Work out the finished part from the listing and answer in its coordinate system (mm). Coordinates: 2 decimals unless noted, no trailing zeros. Loops run counter-clockwise (first coordinate to the right, second up) from the corner with the lowest first, then second, coordinate; pieces in that order, holes last. Notation, with made-up numbers: (87, 44) - (141, 44) arc R29 ccw to (141, 67) - close; hole circle Ø9 at (-3, -4). An arc over 180 degrees is marked (long way). Write each question's results on one line, items separated by ' | '. Start each with the question number.
1. Find the intervals of material crossed by line 1 along X through (y, z) = (1.15, 17.5); line 2 along X through (y, z) = (0.75, 2); line 3 along Z through (x, y) = (20, 2.25), in increasing order. Write a range as [from, to].
2. A cutting plane is placed at B-B on y = 1.8. Determine the outline of the cut face in (x, z).
3. A cutting plane is placed at D-D on z = -17. Determine the outline of the cut face in (x, y).
4. A cutting plane is placed at A-A on z = 17.5. Determine the outline of the cut face in (x, y).
5. A cutting plane is placed at C-C on x = -20. Determine the outline of the cut face in (y, z).
6. This flat-tipped pin is pushed along its axis until it touches: P1, Ø0.9, axis at x = 20.5, y = 1.5, coming from the -Z side. Where does it stop, or does it pass through?
from build123d import *

# Parameters (mm, degrees)
SKETCH_1_W          = 50
SKETCH_1_H          = 55
EXTRUDE_1_DEPTH     = 3
SKETCH_2_R          = 4
CUT_EXTRUDE_1_DEPTH = 3
SKETCH_3_R          = 2
CUT_EXTRUDE_2_DEPTH = 3
SKETCH_4_W          = 3
SKETCH_4_H          = 10
CUT_EXTRUDE_3_DEPTH = 3
CHAMFER_1_SIZE      = 30
CHAMFER_1_SIZE2     = 21.006226146
FILLET_2_R          = 10
FILLET_3_R          = 5


with BuildPart() as part:
    # 草图1 → 凸台-拉伸1 (new body)
    with BuildSketch(Plane(origin=(0, 0, 0), x_dir=(1, 0, 0), z_dir=(0, 1, 0))):
        Rectangle(SKETCH_1_W, SKETCH_1_H)
    extrude(amount=EXTRUDE_1_DEPTH)

    # 草图2 → 切除-拉伸1 (cut)
    with BuildSketch(Plane(origin=(0, 3, 0), x_dir=(1, 0, 0), z_dir=(0, 1, 0))):
        with Locations(Location((4, 17, 0), (0, 0, 270))):
            Circle(SKETCH_2_R)
    extrude(amount=-CUT_EXTRUDE_1_DEPTH, mode=Mode.SUBTRACT)

    # 草图3 → 切除-拉伸2 (cut)
    with BuildSketch(Plane(origin=(0, 3, 0), x_dir=(1, 0, 0), z_dir=(0, 1, 0))):
        with Locations(Location((-20, -17.5, 0), (0, 0, 270))):
            Circle(SKETCH_3_R)
        with Locations(Location((0, -17.5, 0), (0, 0, 270))):
            Circle(SKETCH_3_R)
        with Locations(Location((20, -17.5, 0), (0, 0, 90))):
            Circle(SKETCH_3_R)
    extrude(amount=-CUT_EXTRUDE_2_DEPTH, mode=Mode.SUBTRACT)

    # 草图4 → 切除-拉伸3 (cut)
    with BuildSketch(Plane(origin=(0, 3, 0), x_dir=(1, 0, 0), z_dir=(0, 1, 0))):
        with Locations((-20.5, -2.5)):
            Rectangle(SKETCH_4_W, SKETCH_4_H)
        with Locations((20.5, -2.5)):
            Rectangle(SKETCH_4_W, SKETCH_4_H)
        with Locations((20.5, 17.5)):
            Rectangle(SKETCH_4_W, SKETCH_4_H)
    extrude(amount=-CUT_EXTRUDE_3_DEPTH, mode=Mode.SUBTRACT)

    # 倒角1
    chamfer_1_edges = [part.edges().sort_by_distance(p)[0] for p in [
        (-25, 1.5, -27.5),
    ]]
    chamfer_1_side = [part.faces().sort_by_distance(p)[0] for p in [
        (0, 1.5, -27.5),
    ]]
    chamfer(chamfer_1_edges, length=CHAMFER_1_SIZE, length2=CHAMFER_1_SIZE2, reference=chamfer_1_side[0])

    # 圆角2
    fillet_2_edges = [part.edges().sort_by_distance(p)[0] for p in [
        (-25, 1.5, -6.493773854),
        (5, 1.5, -27.5),
    ]]
    fillet(fillet_2_edges, radius=FILLET_2_R)

    # 圆角3
    fillet_3_edges = [part.edges().sort_by_distance(p)[0] for p in [
        (25, 1.5, -27.5),
    ]]
    fillet(fillet_3_edges, radius=FILLET_3_R)


solid = part.part
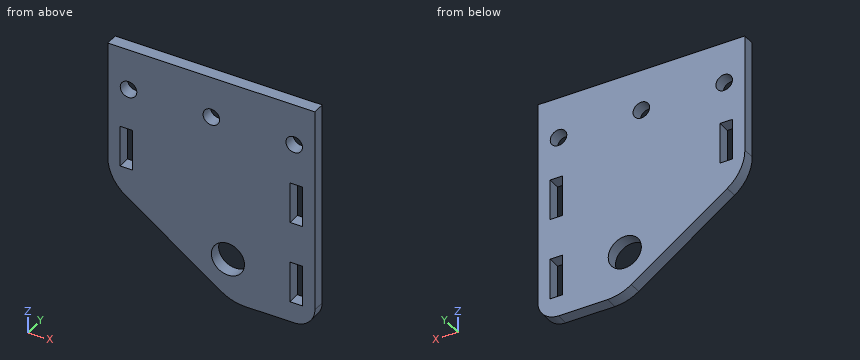
Values:
1) line 1: [-25, -22], [-18, -2], [2, 18], [22, 25] | line 2: [-25, -22], [-19, 19], [22, 25] | line 3: [-27.5, -22.5], [-12.5, -2.5], [7.5, 15.5], [19.5, 27.5]
2) outline: (-25, -1.29) arc R10 ccw to (-20.74, -9.48) - (2.42, -25.69) arc R10 ccw to (8.15, -27.5) - (20, -27.5) arc R5 ccw to (25, -22.5) - (25, 27.5) - (-25, 27.5) - close; hole (-22, -2.5) - (-19, -2.5) - (-19, 7.5) - (-22, 7.5) - close; hole circle Ø4 at (-20, 17.5); hole circle Ø4 at (0, 17.5); hole circle Ø8 at (4, -17); hole circle Ø4 at (20, 17.5); hole (19, -22.5) - (22, -22.5) - (22, -12.5) - (19, -12.5) - close; hole (19, -2.5) - (22, -2.5) - (22, 7.5) - (19, 7.5) - close
3) outline: (-10, 0) - (0, 0) - (0, 3) - (-10, 3) - close; (8, 0) - (19, 0) - (19, 3) - (8, 3) - close; (22, 0) - (25, 0) - (25, 3) - (22, 3) - close
4) outline: (-25, 0) - (-22, 0) - (-22, 3) - (-25, 3) - close; (-18, 0) - (-2, 0) - (-2, 3) - (-18, 3) - close; (2, 0) - (18, 0) - (18, 3) - (2, 3) - close; (22, 0) - (25, 0) - (25, 3) - (22, 3) - close
5) outline: (0, -9.99) - (3, -9.99) - (3, -2.5) - (0, -2.5) - close; (0, 7.5) - (3, 7.5) - (3, 15.5) - (0, 15.5) - close; (0, 19.5) - (3, 19.5) - (3, 27.5) - (0, 27.5) - close
6) P1: z = -27.5
